Read the model definition and answer for the solid it produces. Units are mm, in the model's axes. Coordinates: 2 decimals unless noted, no trailing zeros. Return JSON: item names as keys, results as strings.
Autodesk Inventor part; units mm, degrees
ref_plane "YZ Plane" through (0, 0, 0) normal (1, 0, 0) x (0, 1, 0)
ref_plane "XZ Plane" through (0, 0, 0) normal (0, 1, 0) x (-1, 0, 0)
ref_plane "XY Plane" through (0, 0, 0) normal (0, 0, 1) x (1, 0, 0)
sketch "Sketch1" plane through (0, 0, 0) normal (0, 1, 0) x (-1, 0, 0)
  line L0 (0, 0) -> (485, 0)
  line L1 (485, 0) -> (485, -415)
  line L2 (485, -415) -> (0, -415)
  line L3 (0, -415) -> (0, 0)
  line L4 (485, -207.5) -> (0, -207.5)
  line L5 (0, -207.5) -> (0, 0)
  line L6 (0, -103.75) -> (100, -103.75)
  line L7 (485, -103.75) -> (385, -103.75)
  line L8 (242.5, 0) -> (242.5, -103.75)
  line L9 (242.5, -207.5) -> (242.5, -157.5)
  ellipse E0 centre (242.5, -103.75) end of major axis (385, -103.75) minor radius 53.75
  ellipse E1 centre (242.5, -311.25) end of major axis (385, -311.25) minor radius 53.75
  dimension "d0" = 485
  dimension "d1" = 415
  dimension "d2" = 100
  dimension "d3" = 100
  dimension "d4" = 103.75
  dimension "d5" = 50
  dimension "d6" = 103.75
  dimension "d7" = 103.75
extrude "Extrusion1" add sketch "Sketch1" along normal blind 5 contours L0 L8 E0 L6 L3 | L0 L1 L7 E0 L8 | L6 E0 L9 L4 L3 | L4 L1 L2 L3 | L1 L4 L9 E0 L7
sketch "Sketch2" plane through (0, 5, 0) normal (0, 1, 0) x (1, 0, 0)
  line L0 (0, 0) -> (0, 415)
  line L1 (0, 207.5) -> (0, 209.75)
  line L2 (0, 209.75) -> (0, 207.5)
  line L3 (-485, 0) -> (0, 0)
  line L4 (-242.5, 0) -> (-242.5, 207.5)
  line L5 (0, 209.75) -> (-242.5, 209.75)
  line L6 (-242.5, 209.75) -> (-242.5, 205.25)
  line L7 (-242.5, 205.25) -> (0, 205.25)
  line L8 (0, 205.25) -> (0, 209.75)
  point P0 (0, 205.25)
  dimension "d10" = 2.25
  dimension "d11" = 4.5
extrude "Extrusion2" cut sketch "Sketch2" against normal blind 5 contours L7 L4 L6 L5 L0
sketch "Sketch3" plane through (-485, 0, 0) normal (0, 0, 1) x (1, 0, 0)
  line L0 (485, 0) -> (0, 0)
  line L1 (485, 0) -> (485, 5)
  line L2 (0, 0) -> (485, 0)
  line L3 (485, 0) -> (485, 5)
  line L4 (485, 5) -> (0, 5)
  line L5 (0, 5) -> (0, 0)
extrude "Extrusion3" add sketch "Sketch3" along normal blind 15
sketch "Sketch4" plane through (0, 0, -415) normal (0, 0, -1) x (-1, 0, 0)
  line L0 (485, 0) -> (485, 5)
  line L1 (485, 5) -> (0, 5)
  line L2 (0, 5) -> (0, 0)
  line L3 (0, 0) -> (485, 0)
  line L4 (485, 0) -> (485, 5)
extrude "Extrusion4" add sketch "Sketch4" along normal blind 15
sketch "Sketch5" plane through (0, 5, 0) normal (0, 1, 0) x (1, 0, 0)
  line L0 (-485, -15) -> (-485, 430)
  line L1 (-485, 207.5) -> (54.8472, 207.5)
  line L2 (-485, 0) -> (-460, 0)
  line L3 (-460, 0) -> (-460, 4.5)
  line L4 (-460, 4.5) -> (-485, 4.5)
  line L5 (-485, 4.5) -> (-485, 0)
  line L6 (0, 0) -> (-85, 0)
  line L7 (-85, 0) -> (-85, 4.5)
  line L8 (-85, 4.5) -> (0, 4.5)
  line L9 (0, 4.5) -> (0, 0)
  line L10 (0, -15) -> (-485, -15)
  line L11 (-485, 415) -> (-460, 415)
  line L12 (-460, 415) -> (-460, 410.5)
  line L13 (-460, 410.5) -> (-485, 410.5)
  line L14 (-485, 410.5) -> (-485, 415)
  line L15 (0, 415) -> (-85, 415)
  line L16 (-85, 415) -> (-85, 410.5)
  line L17 (-85, 410.5) -> (0, 410.5)
  line L18 (0, 410.5) -> (0, 415)
  line L19 (0, 205.25) -> (-242.5, 205.25)
  line L20 (-242.5, 205.25) -> (-242.5, 207.5)
  line L21 (-242.5, 205.25) -> (-242.5, 209.75)
  dimension "d18" = 25
  dimension "d19" = 4.5
  dimension "d20" = 85
  dimension "d21" = 4.5
  dimension "d22" = 15
extrude "Extrusion5" cut sketch "Sketch5" against normal blind 5
sketch "Sketch6" plane through (0, 5, 0) normal (0, 1, 0) x (1, 0, 0)
  line L0 (-15, 4.5) -> (-15, 584.4984)
  line L1 (-15, 4.5) -> (-15, 48.5)
  line L2 (-15, 48.5) -> (0, 48.5)
  line L3 (0, 48.5) -> (0, 53)
  line L4 (0, 53) -> (-15, 53)
  line L5 (-15, 53) -> (-15, 48.5)
  line L6 (-15, 100.75) -> (0, 100.75)
  line L7 (0, 100.75) -> (0, 105.25)
  line L8 (0, 105.25) -> (-15, 105.25)
  line L9 (-15, 105.25) -> (-15, 100.75)
  line L10 (-15, 153) -> (0, 153)
  line L11 (0, 153) -> (0, 157.5)
  line L12 (0, 157.5) -> (-15, 157.5)
  line L13 (-15, 157.5) -> (-15, 153)
  line L14 (-15, 205.25) -> (0, 205.25)
  line L15 (0, 205.25) -> (0, 209.75)
  line L16 (0, 209.75) -> (-15, 209.75)
  line L17 (-15, 209.75) -> (-15, 205.25)
  line L18 (-15, 257.5) -> (0, 257.5)
  line L19 (0, 257.5) -> (0, 262)
  line L20 (0, 262) -> (-15, 262)
  line L21 (-15, 262) -> (-15, 257.5)
  line L22 (-15, 309.75) -> (0, 309.75)
  line L23 (0, 309.75) -> (0, 314.25)
  line L24 (0, 314.25) -> (-15, 314.25)
  line L25 (-15, 314.25) -> (-15, 309.75)
  line L26 (-15, 362) -> (0, 362)
  line L27 (0, 362) -> (0, 366.5)
  line L28 (0, 366.5) -> (-15, 366.5)
  line L29 (-15, 366.5) -> (-15, 362)
  line L30 (0, 205.25) -> (0, 4.5)
  line L31 (0, 4.5) -> (-15, 4.5)
  line L32 (0, 4.5) -> (-85, 4.5)
  line L33 (0, 209.75) -> (0, 410.5)
  point P0 (0, 0)
  point P1 (-15, 53)
  point P2 (-15, 100.75)
  point P3 (-15, 105.25)
  point P4 (-15, 262)
  point P5 (-15, 257.5)
  point P6 (-15, 314.25)
  point P7 (-15, 309.75)
  point P8 (-15, 366.5)
  point P9 (-15, 362)
  dimension "d29" = 44
  dimension "d30" = 15
  dimension "d31" = 4.5
  dimension "d32" = 52.25
  dimension "d34" = 15
  dimension "d35" = 0
extrude "Extrusion6" cut sketch "Sketch6" against normal blind 5 contours L0 L4 L3 L2 | L0 L8 L7 L6 | L0 L12 L11 L10 | L0 L20 L19 L18 | L0 L24 L23 L22 | L0 L28 L27 L26
fillet "Fillet1" radius 1 45 edges at (-460, 2.5, 0) (-460, 2.5, -4.5) (-485, 2.5, -4.5) (-485, 2.5, 0) (-485, 2.5, 15) (0, 2.5, 15) (-85, 2.5, -4.5) (-85, 2.5, 0) (0, 2.5, -4.5) (-15, 2.5, -53) (-15, 2.5, -48.5) (-15, 2.5, -105.25) (-15, 2.5, -100.75) (0, 2.5, -100.75) (0, 2.5, -105.25) (-15, 2.5, -157.5) (-15, 2.5, -153) (0, 2.5, -153) (0, 2.5, -157.5) (0, 2.5, -205.25) (0, 2.5, -209.75) (-242.5, 2.5, -209.75) (-242.5, 2.5, -205.25) (0, 2.5, -257.5) (0, 2.5, -262) (-15, 2.5, -262) (-15, 2.5, -257.5) (0, 2.5, -309.75) (0, 2.5, -314.25) (-15, 2.5, -314.25) (-15, 2.5, -309.75) (-15, 2.5, -366.5) (-15, 2.5, -362) (0, 2.5, -362) (0, 2.5, -366.5) (0, 2.5, -415) (0, 2.5, -410.5) (0, 2.5, -430) (-85, 2.5, -415) (-85, 2.5, -410.5) (-460, 2.5, -410.5) (-460, 2.5, -415) (-485, 2.5, -430) (-485, 2.5, -415) (-485, 2.5, -410.5)
properties part number "inside_leg_2" material "Foam Core Board"
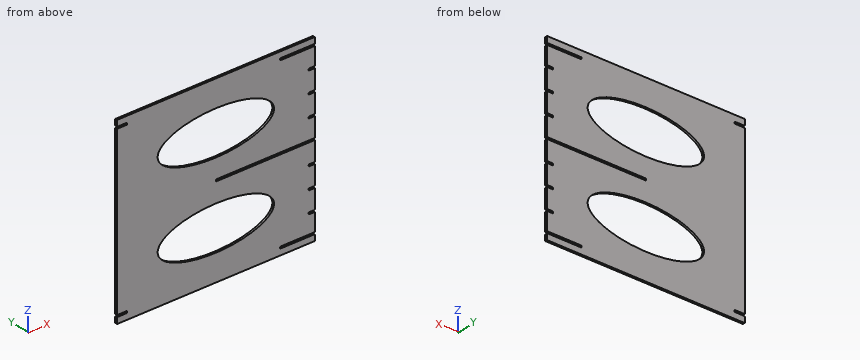
(1) A cutting plane is placed at A-A (y = 3.6). State how many separate pieces and enclosed holes the cut face has, and give its area (3 significant figures).
Answer:
{"separate pieces": "1", "enclosed holes": "2", "area": "165,000 mm²"}
(2) Straight lines are drawn through the part: line 1 (Z direction, x = -184, y = 1.45); line 2 (Z direction, x = -318, y = 1.45); line 3 (Z direction, x = -301, y = 0.9). For each, find the intervals that lie inside material, in ascending order. Write a range as from..to.
Answer:
{"line 1": "-430..-360.26, -262.24..-209.75, -205.25..-152.76, -54.74..15", "line 2": "-430..-356.84, -265.66..-149.34, -58.16..15", "line 3": "-430..-360.26, -262.24..-152.76, -54.74..15"}
(3) Flat-ended cylindrical pins translate along their axes: P1, Ø2, axis at y = 3.5, z = -51, coming from the +X side; P2, Ø1.2, axis at y = 2.5, z = -413.5, coming from the +X side (3 decimals); P3, Ø3, axis at y = 3, z = -207, coming from the +X side. Find the tip coordinate at first contact, or state that the pin passes through.
Answer:
{"P1": "x = -15", "P2": "x = -84.995", "P3": "x = -242.16"}
